Input: part model. Units: mm. Frame: model coordinates. Face numbers are marked on the shaded views. A direction names the side the tool comes from. Coordinates: 2 decimals unless noted, no trailing zeros. Write each loop counter-clockwise with the first axis right and the second up, starting at its lowest first coordinate (ties: lowest second). Pieces come first, ordered by that corner, then holes. Notation, with made-up numbers: (10, -29.5) - (66, -29.5) arc R29 ccw to (66, 9.5) - close; hole circle Ø10 at (-29, 3.25). An arc over 180 degrees is marked (long way). Put each result on its own line as item: value. Start each with the question number.
1. Pull-direction query (Y, two-part tool) for the marked faces 1, 2 and 3; classes: released by +Y, released by -Y, zero draft, split by the parting line, or undercut.
2. Cut plane B-B, the plane z = -13. Return loops of the section in (x, y).
3. Pin query (flat end, axial travel): pin 1 (6 mm diameter, centred on x = 2, y = -3, fed in from +Z); pin 2 (1.6 mm diameter, centred on y = 13, z = 23.5, fed in from +X); pin 3 (1 mm diameter, centred on x = 6, z = 19, fed in from -Y). Return the tip coordinate at first contact, or that it passes through.
4. Cut plane A-A, the plane y = -10.25. Return loops of the section in (x, z), and give its area (3 significant figures).
5. Line query: line 1 (Y direction, x = 0, z = -25.4); line 2 (Z direction, x = 1.5, y = -12.5); line 3 (Z direction, x = -7, y = 3.75). Output: solid intervals per line, ascending.
6. Access query for the marked faces 4, 5 and 6. Directions: +Z, -Z, +X, -X, +Y, -Y. A direction counts if a zero-diameter tool reaches every point of the face in a straight line with its end or side. Return the directions, or none.
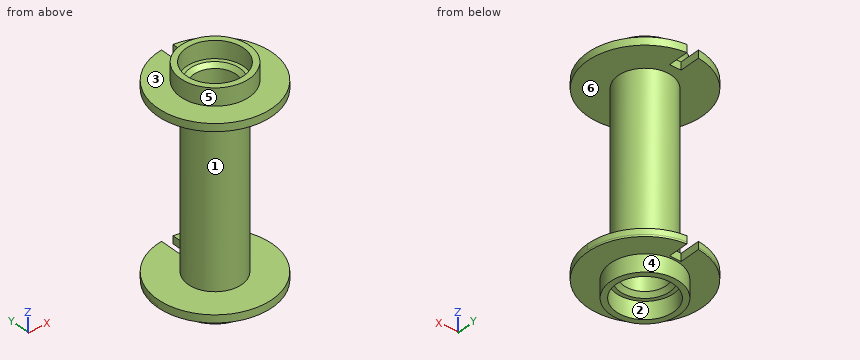
from build123d import *

# Parameters (mm, degrees)
SKETCH_1_R             = 7
SKETCH_1_R_2           = 5.5
EXTRUDE_1_DEPTH        = 29.5
EXTRUDE_START          = -7
SKETCH_2_R             = 15
SKETCH_2_R_2           = 5.5
EXTRUDE_2_DEPTH        = 7
SKETCH_5_W             = 5.5
SKETCH_5_H             = 9
CUT_EXTRUDE_4_DEPTH    = 15
HOLE_WIZARD_M3_1_D     = 2.5
HOLE_WIZARD_M3_1_DEPTH = 9.5
HOLE_WIZARD_M3_1_TIP   = 0.751075774
CHAMFER_1_SIZE         = 0.5
CHAMFER_2_SIZE         = 2
SKETCH1_R              = 7.5
EXTRUDE1_DEPTH         = 5
SKETCH2_W              = 25
SKETCH2_H              = 6
EXTRUDE2_DEPTH         = 5.5
CHAMFER2_SIZE          = 2
SKETCH4_R              = 17.5
EXTRUDE3_DEPTH         = 5.5
SKETCH5_R              = 17.5
EXTRUDE4_DEPTH         = 5.5
SKETCH6_R              = 9
SKETCH6_R_2            = 7.5
EXTRUDE5_DEPTH         = 5
SKETCH7_R              = 15
SKETCH7_R_2            = 5.5
EXTRUDE6_DEPTH         = 0.5
EXTRUDE7_START         = 0.5
SKETCH8_R              = 15
SKETCH8_R_2            = 5.5
EXTRUDE7_DEPTH         = 0.5
CHAMFER3_SIZE          = 1
EXTRUDE10_REACH        = 59.552
SKETCH11_W             = 3
SKETCH11_H             = 5.5


with BuildPart() as part:
    # 草图1 → 拉伸1 (new, symmetric)
    with BuildSketch(Plane.XY):
        Circle(SKETCH_1_R)
        Circle(SKETCH_1_R_2, mode=Mode.SUBTRACT)
    extrude(amount=EXTRUDE_1_DEPTH, both=True)

    # 草图2 → 拉伸2 (add)
    with BuildSketch(Plane.XY.offset(29.5).offset(EXTRUDE_START)):
        Circle(SKETCH_2_R)
        Circle(SKETCH_2_R_2, mode=Mode.SUBTRACT)
    extrude_2 = extrude(amount=EXTRUDE_2_DEPTH)

    # 镜向1: 拉伸2 across plane
    add(extrude_2.mirror(Plane.XY))

    # 草图5 → 拉伸4 (cut, symmetric)
    with BuildSketch(Plane(origin=(0, 0, 0), x_dir=(0, 0, -1), z_dir=(1, 0, 0))):
        with Locations((-26.75, -15.5)):
            Rectangle(SKETCH_5_W, SKETCH_5_H)
        with Locations((26.75, -15.5)):
            Rectangle(SKETCH_5_W, SKETCH_5_H)
    extrude(amount=CUT_EXTRUDE_4_DEPTH, both=True, mode=Mode.SUBTRACT)

    # M3 螺纹孔1
    with Locations(Plane(origin=(-8, -11, 27.5), x_dir=(0, 0, -1), z_dir=(0, -1, 0))):
        with Locations((0, 0), (0, 16), (55, 0), (55, 16)):
            Hole(HOLE_WIZARD_M3_1_D / 2, depth=HOLE_WIZARD_M3_1_DEPTH)
            with Locations((0, 0, -(HOLE_WIZARD_M3_1_DEPTH + HOLE_WIZARD_M3_1_TIP / 2))):  # 118° drill point
                Cone(0, HOLE_WIZARD_M3_1_D / 2, HOLE_WIZARD_M3_1_TIP, mode=Mode.SUBTRACT)

    # 倒角1
    chamfer_1_edges = [part.edges().sort_by_distance(p)[0] for p in [
        (8, -11, -28.75),
        (-8, -11, -28.75),
        (8, -11, 26.25),
        (-8, -11, 26.25),
    ]]
    chamfer(chamfer_1_edges, length=CHAMFER_1_SIZE)

    # 倒角2
    chamfer_2_edges = [part.edges().sort_by_distance(p)[0] for p in [
        (-5.5, 0, -29.5),
    ]]
    chamfer(chamfer_2_edges, length=CHAMFER_2_SIZE)

    # Sketch1 → Extrude1 (cut)
    with BuildSketch(Plane(origin=(0, 0, 29.5), x_dir=(-1, 0, 0), z_dir=(0, 0, -1))):
        Circle(SKETCH1_R)
    extrude(amount=EXTRUDE1_DEPTH, mode=Mode.SUBTRACT)

    # Sketch2 → Extrude2 (cut)
    with BuildSketch(Plane.XY.offset(-29.5)):
        with Locations((0, 12)):
            Rectangle(SKETCH2_W, SKETCH2_H)
    extrude(amount=EXTRUDE2_DEPTH, mode=Mode.SUBTRACT)

    # Chamfer2
    # the kernel refuses this chamfer: 2 mm, written as the material it takes off along each edge
    with BuildSketch(Plane(origin=(0, 0, 29.5), x_dir=(-1, 0, 0), z_dir=(0, -1, 0))) as chamfer2_piece_1:
        Polygon((7.5, CHAMFER2_SIZE), (7.5 + CHAMFER2_SIZE, 0), (7.5, 0), align=None)
    revolve(axis=Axis((0, 0, 29.5), (0, 0, -1)), mode=Mode.SUBTRACT)

    # Sketch4 → Extrude3 (cut)
    with BuildSketch(Plane.XY.offset(29.5)):
        Circle(SKETCH4_R)
    extrude(amount=-EXTRUDE3_DEPTH, mode=Mode.SUBTRACT)

    # Sketch5 → Extrude4 (cut)
    with BuildSketch(Plane(origin=(0, 0, -29.5), x_dir=(-1, 0, 0), z_dir=(0, 0, -1))):
        Circle(SKETCH5_R)
    extrude(amount=-EXTRUDE4_DEPTH, mode=Mode.SUBTRACT)

    # Sketch6 → Extrude5 (add)
    with BuildSketch(Plane.XY.offset(24)):
        with Locations(Location((0, 0, 0), (0, 0, 180))):
            Circle(SKETCH6_R)
        Circle(SKETCH6_R_2, mode=Mode.SUBTRACT)
    extrude5 = extrude(amount=EXTRUDE5_DEPTH)

    # Mirror1: Extrude5 across plane
    add(extrude5.mirror(Plane.XY))

    # Sketch7 → Extrude6 (add)
    with BuildSketch(Plane.XY.offset(24)):
        Circle(SKETCH7_R)
        Circle(SKETCH7_R_2, mode=Mode.SUBTRACT)
    extrude(amount=EXTRUDE6_DEPTH)

    # Sketch8 → Extrude7 (add)
    with BuildSketch(Plane(origin=(0, 0, -24), x_dir=(-1, 0, 0), z_dir=(0, 0, -1)).offset(EXTRUDE7_START)):
        Circle(SKETCH8_R)
        Circle(SKETCH8_R_2, mode=Mode.SUBTRACT)
    extrude(amount=-EXTRUDE7_DEPTH)

    # Chamfer3
    # the kernel refuses this chamfer: 1 mm, written as the material it takes off along each edge
    with BuildSketch(Plane(origin=(0, 0, 24.5), x_dir=(1, 0, 0), z_dir=(0, -1, 0))) as chamfer3_piece_1:
        Polygon((5.5, -CHAMFER3_SIZE), (5.5 + CHAMFER3_SIZE, 0), (5.5, 0), align=None)
    revolve(axis=Axis((0, 0, 24.5), (0, 0, 1)), mode=Mode.SUBTRACT)
    with BuildSketch(Plane(origin=(0, 0, -24.5), x_dir=(-1, 0, 0), z_dir=(0, -1, 0))) as chamfer3_piece_2:
        Polygon((5.5 + CHAMFER3_SIZE, 0), (5.5, -CHAMFER3_SIZE), (5.5, 0), align=None)
    revolve(axis=Axis((0, 0, -24.5), (0, 0, -1)), mode=Mode.SUBTRACT)

    # Extrude10: up to this face of the body (flat: up to its plane)
    extrude10_end = Plane(part.part.faces().sort_by_distance((14.575735931, 0, -24.5))[0])
    # Sketch11 → Extrude10 (cut, up to the picked face)
    with BuildSketch(Plane.XY.offset(24.5), mode=Mode.PRIVATE) as extrude10_sk1:
        with Locations((0, 12.25)):
            Rectangle(SKETCH11_W, SKETCH11_H)
    extrude10_tool1 = split(extrude(extrude10_sk1.sketch, amount=-EXTRUDE10_REACH, mode=Mode.PRIVATE), bisect_by=extrude10_end, keep=Keep.BOTH, mode=Mode.PRIVATE)
    add(extrude10_tool1.solids().sort_by(Axis((0, 12.25, 24.5), (0, 0, -1)))[0], mode=Mode.SUBTRACT)


solid = part.part
Report:
1. face 1: split by the parting line
1. face 2: undercut
1. face 3: zero draft
2. outline: circle Ø14 at (0, 0); hole circle Ø11 at (0, 0)
3. pin 1: stops at z = 24.5
3. pin 2: stops at x = 8.73
3. pin 3: stops at y = -4.33
4. outline: (-10.95, -24.5) - (10.95, -24.5) - (10.95, -22.5) - (-10.95, -22.5) - close; (-10.95, 22.5) - (10.95, 22.5) - (10.95, 24.5) - (-10.95, 24.5) - close
4. area: 87.6 mm^2
5. line 1: y = -9 to -7.5, 7.5 to 9
5. line 2: z = -24.5 to -22.5, 22.5 to 24.5
5. line 3: z = -29 to -22.5, 22.5 to 29
6. face 4: -Z
6. face 5: +Z
6. face 6: none
